Verification items for the finished model (mm, model axes). Face numbers are marked on the shaded views. A direction names the side the tool comes from. Round coordinates to 2 decimals unless told otherwise and drop trailing zeros. Loops run counter-clockwise (first coordinate to the right, second up) from the corner with the lowest first, then second, coordinate; pieces in that order, holes last. Notation, with made-up numbers: M 33.5,36 L 85.5,36 A20 cw 85.5,50 Z; hole C 26,58 d2. An arc over 180 degrees is marked long. One line per item, written item: value.
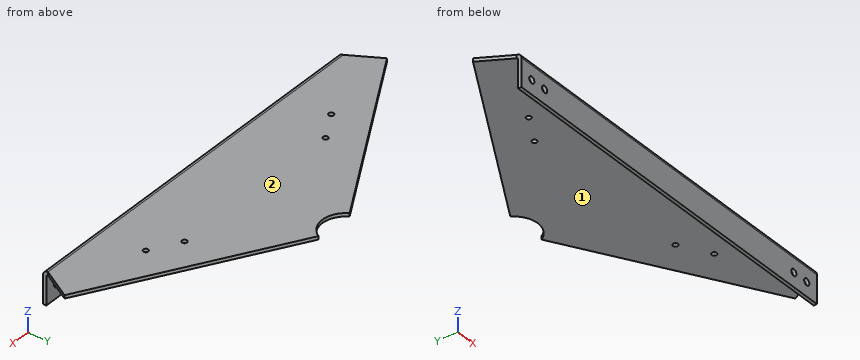
from build123d import *

# Parameters (mm, degrees)
SKETCH_10_R                   = 10
SM_BASE_FLANGE_3_DEPTH        = 2
SM_EDGE_FLANGE_6_DEPTH        = 230
SM_EDGE_FLANGE_6_BEND_DEPTH   = 230
SM_EDGE_FLANGE_6_BEND_2_DEPTH = 230
CUT_EXTRUDE_4_REACH           = 363.137
SKETCH_47_R                   = 2
CUT_EXTRUDE_6_REACH           = 263.424
SKETCH_50_R                   = 2
CUT_EXTRUDE_7_REACH           = 351.772
SKETCH_51_R                   = 2
CUT_EXTRUDE_8_REACH           = 349.61
SKETCH_52_R                   = 14
SKETCH_53_R                   = 1.5
CUT_EXTRUDE_9_DEPTH           = 10
OTHER_START                   = -20
OTHER_1_OUTLINE_R             = 1.5
OTHER_1_OUTLINE_R_2           = 10
OTHER_1_DEPTH                 = 20


# Read off the part's stored shape, not the designer's step: Полость1
# Sheet-metal steps are written as plain solids
with BuildPart() as part:
    # Эскиз10 → Базовая кромка3 (new body)
    with BuildSketch(Plane.XY):
        Polygon((0, 0), (-21, 36.373066959), (94, 235.558909829), (136, 235.558909829), (251, 36.373066959), (230, 0), align=None)
        with Locations((171.849364905, 123.465988394)):
            Circle(SKETCH_10_R, mode=Mode.SUBTRACT)
    extrude(amount=-SM_BASE_FLANGE_3_DEPTH)

    # Ребро-кромка6 section (across the edge) → Ребро-кромка6 (add)
    with BuildSketch(Plane(origin=(-21.866025404, 36.873066959, -2), x_dir=(0.8660254037844436, -0.4999999999999914, -3.4914813388431334e-15), z_dir=(0.4999999999999914, 0.8660254037844436, 0))):
        with BuildLine():
            Line((-2, 1), (-2, 18))
            Line((-2, 18), (0, 18))
            Line((0, 18), (0, 1))
            ThreePointArc((0, 1), (0.292893219, 0.292893219), (1, 0))
            Line((1, 0), (1, -2))
            ThreePointArc((1, -2), (-1.121320344, -1.121320344), (-2, 1))
        make_face()
    extrude(amount=SM_EDGE_FLANGE_6_DEPTH)

    # Ребро-кромка6 section 2 (across the edge) → Ребро-кромка6 bend (add)
    with BuildSketch(Plane(origin=(136.866025404, 236.058909829, -2), x_dir=(-0.8660254037844363, -0.5000000000000041, -3.4914813388431334e-15), z_dir=(0.5000000000000041, -0.8660254037844363, 0))):
        with BuildLine():
            Line((-2, 1), (-2, 18))
            Line((-2, 18), (0, 18))
            Line((0, 18), (0, 1))
            ThreePointArc((0, 1), (0.292893219, 0.292893219), (1, 0))
            Line((1, 0), (1, -2))
            ThreePointArc((1, -2), (-1.121320344, -1.121320344), (-2, 1))
        make_face()
    extrude(amount=SM_EDGE_FLANGE_6_BEND_DEPTH)

    # Ребро-кромка6 section 3 (across the edge) → Ребро-кромка6 bend 2 (add)
    with BuildSketch(Plane(origin=(230, -1, -2), x_dir=(0, 1, 0), z_dir=(-1, 0, 0))):
        with BuildLine():
            Line((-2, 1), (-2, 18))
            Line((-2, 18), (0, 18))
            Line((0, 18), (0, 1))
            ThreePointArc((0, 1), (0.292893219, 0.292893219), (1, 0))
            Line((1, 0), (1, -2))
            ThreePointArc((1, -2), (-1.121320344, -1.121320344), (-2, 1))
        make_face()
    extrude(amount=SM_EDGE_FLANGE_6_BEND_2_DEPTH)

    # Эскиз47 → Вырез-Вытянуть4 (cut, up to next)
    with BuildSketch(Plane(origin=(-34.098076211, 19.686533479, 0), x_dir=(0, 0, 1), z_dir=(-0.866025403784443, 0.4999999999999925, 3.788649256556814e-15)), mode=Mode.PRIVATE) as cut_extrude_4_sk1:
        with Locations(Location((-11.5, 29, 0), (0, 0, 270))):
            Circle(SKETCH_47_R)
    cut_extrude_4_tool1 = extrude(cut_extrude_4_sk1.sketch, amount=-CUT_EXTRUDE_4_REACH, mode=Mode.PRIVATE) & part.part
    # Эскиз47 → Вырез-Вытянуть4 (cut, up to next)
    with BuildSketch(Plane(origin=(-34.098076211, 19.686533479, 0), x_dir=(0, 0, 1), z_dir=(-0.866025403784443, 0.4999999999999925, 3.788649256556814e-15)), mode=Mode.PRIVATE) as cut_extrude_4_sk2:
        with Locations(Location((-11.5, 39, 0), (0, 0, 270))):
            Circle(SKETCH_47_R)
    cut_extrude_4_tool2 = extrude(cut_extrude_4_sk2.sketch, amount=-CUT_EXTRUDE_4_REACH, mode=Mode.PRIVATE) & part.part
    # Эскиз47 → Вырез-Вытянуть4 (cut, up to next)
    with BuildSketch(Plane(origin=(-34.098076211, 19.686533479, 0), x_dir=(0, 0, 1), z_dir=(-0.866025403784443, 0.4999999999999925, 3.788649256556814e-15)), mode=Mode.PRIVATE) as cut_extrude_4_sk3:
        with Locations(Location((-11.5, 233, 0), (0, 0, 270))):
            Circle(SKETCH_47_R)
    cut_extrude_4_tool3 = extrude(cut_extrude_4_sk3.sketch, amount=-CUT_EXTRUDE_4_REACH, mode=Mode.PRIVATE) & part.part
    # Эскиз47 → Вырез-Вытянуть4 (cut, up to next)
    with BuildSketch(Plane(origin=(-34.098076211, 19.686533479, 0), x_dir=(0, 0, 1), z_dir=(-0.866025403784443, 0.4999999999999925, 3.788649256556814e-15)), mode=Mode.PRIVATE) as cut_extrude_4_sk4:
        with Locations(Location((-11.5, 243, 0), (0, 0, 270))):
            Circle(SKETCH_47_R)
    cut_extrude_4_tool4 = extrude(cut_extrude_4_sk4.sketch, amount=-CUT_EXTRUDE_4_REACH, mode=Mode.PRIVATE) & part.part
    add(cut_extrude_4_tool1.solids().sort_by_distance((-19.598076, 44.80127, -11.5))[0], mode=Mode.SUBTRACT)
    add(cut_extrude_4_tool2.solids().sort_by_distance((-14.598076, 53.461524, -11.5))[0], mode=Mode.SUBTRACT)
    add(cut_extrude_4_tool3.solids().sort_by_distance((82.401924, 221.470453, -11.5))[0], mode=Mode.SUBTRACT)
    add(cut_extrude_4_tool4.solids().sort_by_distance((87.401924, 230.130707, -11.5))[0], mode=Mode.SUBTRACT)

    # Эскиз50 → Вырез-Вытянуть6 (cut, up to next)
    with BuildSketch(Plane(origin=(206.598076211, 119.279454915, 0), x_dir=(0, 0, -1), z_dir=(0.866025403784436, 0.5000000000000047, 3.0623287353932815e-15)), mode=Mode.PRIVATE) as cut_extrude_6_sk1:
        with Locations(Location((11.5, -86, 0), (0, 0, 90))):
            Circle(SKETCH_50_R)
    cut_extrude_6_tool1 = extrude(cut_extrude_6_sk1.sketch, amount=-CUT_EXTRUDE_6_REACH, mode=Mode.PRIVATE) & part.part
    # Эскиз50 → Вырез-Вытянуть6 (cut, up to next)
    with BuildSketch(Plane(origin=(206.598076211, 119.279454915, 0), x_dir=(0, 0, -1), z_dir=(0.866025403784436, 0.5000000000000047, 3.0623287353932815e-15)), mode=Mode.PRIVATE) as cut_extrude_6_sk2:
        with Locations(Location((11.5, -76, 0), (0, 0, 90))):
            Circle(SKETCH_50_R)
    cut_extrude_6_tool2 = extrude(cut_extrude_6_sk2.sketch, amount=-CUT_EXTRUDE_6_REACH, mode=Mode.PRIVATE) & part.part
    # Эскиз50 → Вырез-Вытянуть6 (cut, up to next)
    with BuildSketch(Plane(origin=(206.598076211, 119.279454915, 0), x_dir=(0, 0, -1), z_dir=(0.866025403784436, 0.5000000000000047, 3.0623287353932815e-15)), mode=Mode.PRIVATE) as cut_extrude_6_sk3:
        with Locations(Location((11.5, 118, 0), (0, 0, 90))):
            Circle(SKETCH_50_R)
    cut_extrude_6_tool3 = extrude(cut_extrude_6_sk3.sketch, amount=-CUT_EXTRUDE_6_REACH, mode=Mode.PRIVATE) & part.part
    # Эскиз50 → Вырез-Вытянуть6 (cut, up to next)
    with BuildSketch(Plane(origin=(206.598076211, 119.279454915, 0), x_dir=(0, 0, -1), z_dir=(0.866025403784436, 0.5000000000000047, 3.0623287353932815e-15)), mode=Mode.PRIVATE) as cut_extrude_6_sk4:
        with Locations(Location((11.5, 128, 0), (0, 0, 90))):
            Circle(SKETCH_50_R)
    cut_extrude_6_tool4 = extrude(cut_extrude_6_sk4.sketch, amount=-CUT_EXTRUDE_6_REACH, mode=Mode.PRIVATE) & part.part
    add(cut_extrude_6_tool1.solids().sort_by_distance((249.598076, 44.80127, -11.5))[0], mode=Mode.SUBTRACT)
    add(cut_extrude_6_tool2.solids().sort_by_distance((244.598076, 53.461524, -11.5))[0], mode=Mode.SUBTRACT)
    add(cut_extrude_6_tool3.solids().sort_by_distance((147.598076, 221.470453, -11.5))[0], mode=Mode.SUBTRACT)
    add(cut_extrude_6_tool4.solids().sort_by_distance((142.598076, 230.130707, -11.5))[0], mode=Mode.SUBTRACT)

    # Эскиз51 → Вырез-Вытянуть7 (cut, up to next)
    with BuildSketch(Plane.XZ.offset(3), mode=Mode.PRIVATE) as cut_extrude_7_sk1:
        with Locations(Location((222, -11.5, 0), (0, 0, 270))):
            Circle(SKETCH_51_R)
    cut_extrude_7_tool1 = extrude(cut_extrude_7_sk1.sketch, amount=-CUT_EXTRUDE_7_REACH, mode=Mode.PRIVATE) & part.part
    # Эскиз51 → Вырез-Вытянуть7 (cut, up to next)
    with BuildSketch(Plane.XZ.offset(3), mode=Mode.PRIVATE) as cut_extrude_7_sk2:
        with Locations(Location((212, -11.5, 0), (0, 0, 270))):
            Circle(SKETCH_51_R)
    cut_extrude_7_tool2 = extrude(cut_extrude_7_sk2.sketch, amount=-CUT_EXTRUDE_7_REACH, mode=Mode.PRIVATE) & part.part
    # Эскиз51 → Вырез-Вытянуть7 (cut, up to next)
    with BuildSketch(Plane.XZ.offset(3), mode=Mode.PRIVATE) as cut_extrude_7_sk3:
        with Locations(Location((18, -11.5, 0), (0, 0, 270))):
            Circle(SKETCH_51_R)
    cut_extrude_7_tool3 = extrude(cut_extrude_7_sk3.sketch, amount=-CUT_EXTRUDE_7_REACH, mode=Mode.PRIVATE) & part.part
    # Эскиз51 → Вырез-Вытянуть7 (cut, up to next)
    with BuildSketch(Plane.XZ.offset(3), mode=Mode.PRIVATE) as cut_extrude_7_sk4:
        with Locations(Location((8, -11.5, 0), (0, 0, 270))):
            Circle(SKETCH_51_R)
    cut_extrude_7_tool4 = extrude(cut_extrude_7_sk4.sketch, amount=-CUT_EXTRUDE_7_REACH, mode=Mode.PRIVATE) & part.part
    add(cut_extrude_7_tool1.solids().sort_by_distance((222, -3, -11.5))[0], mode=Mode.SUBTRACT)
    add(cut_extrude_7_tool2.solids().sort_by_distance((212, -3, -11.5))[0], mode=Mode.SUBTRACT)
    add(cut_extrude_7_tool3.solids().sort_by_distance((18, -3, -11.5))[0], mode=Mode.SUBTRACT)
    add(cut_extrude_7_tool4.solids().sort_by_distance((8, -3, -11.5))[0], mode=Mode.SUBTRACT)

    # Эскиз52 → Вырез-Вытянуть8 (cut, up to next)
    with BuildSketch(Plane(origin=(0, 0, -2), x_dir=(-1, 0, 0), z_dir=(0, 0, -1)), mode=Mode.PRIVATE) as cut_extrude_8_sk1:
        with Locations((-115, 90.643992263)):
            Circle(SKETCH_52_R)
    cut_extrude_8_tool1 = extrude(cut_extrude_8_sk1.sketch, amount=-CUT_EXTRUDE_8_REACH, mode=Mode.PRIVATE) & part.part
    add(cut_extrude_8_tool1.solids().sort_by_distance((115, 90.643992, -2))[0], mode=Mode.SUBTRACT)

    # Эскиз53 → Вырез-Вытянуть9 (cut)
    with BuildSketch(Plane(origin=(0, 0, -2), x_dir=(-1, 0, 0), z_dir=(0, 0, -1))):
        with Locations((-40.121778265, 70.507041555)):
            Circle(SKETCH_53_R)
        with Locations((-22.801270189, 60.507041555)):
            Circle(SKETCH_53_R)
        with Locations((-60.121778265, 35.866025404)):
            Circle(SKETCH_53_R)
        with Locations((-42.801270189, 25.866025404)):
            Circle(SKETCH_53_R)
        with Locations((-95, 185.558909829)):
            Circle(SKETCH_53_R)
        with Locations((-95, 165.558909829)):
            Circle(SKETCH_53_R)
        with Locations((-135, 185.558909829)):
            Circle(SKETCH_53_R)
        with Locations((-135, 165.558909829)):
            Circle(SKETCH_53_R)
        with Locations((-207.198729811, 60.507041555)):
            Circle(SKETCH_53_R)
        with Locations((-189.878221735, 70.507041555)):
            Circle(SKETCH_53_R)
        with Locations((-187.198729811, 25.866025404)):
            Circle(SKETCH_53_R)
        with Locations((-169.878221735, 35.866025404)):
            Circle(SKETCH_53_R)
    extrude(amount=-CUT_EXTRUDE_9_DEPTH, mode=Mode.SUBTRACT)

    # Полость1 outline → Полость1 (cut)
    with BuildSketch(Plane.XY.offset(OTHER_START)):
        with BuildLine():
            Line((127.120094671, 83.636617208), (240.495741262, 18.17915713))
            Line((240.495741262, 18.17915713), (251, 36.373066959))
            Line((251, 36.373066959), (253.598076211, 37.873066959))
            Line((253.598076211, 37.873066959), (138.598076211, 237.058909829))
            Line((138.598076211, 237.058909829), (136, 235.558909829))
            Line((136, 235.558909829), (94, 235.558909829))
            Line((94, 235.558909829), (91.401923789, 237.058909829))
            Line((91.401923789, 237.058909829), (-23.598076211, 37.873066959))
            Line((-23.598076211, 37.873066959), (-21, 36.373066959))
            Line((-21, 36.373066959), (-10.495741262, 18.17915713))
            Line((-10.495741262, 18.17915713), (102.879905329, 83.636617208))
            ThreePointArc((102.879905329, 83.636617208), (115, 104.643992263), (127.120094671, 83.636617208))
        make_face()
        with Locations((22.801270189, 60.507041555)):
            Circle(OTHER_1_OUTLINE_R, mode=Mode.SUBTRACT)
        with Locations((40.121778265, 70.507041555)):
            Circle(OTHER_1_OUTLINE_R, mode=Mode.SUBTRACT)
        with Locations((189.878221735, 70.507041555)):
            Circle(OTHER_1_OUTLINE_R, mode=Mode.SUBTRACT)
        with Locations((207.198729811, 60.507041555)):
            Circle(OTHER_1_OUTLINE_R, mode=Mode.SUBTRACT)
        with Locations((171.849364905, 123.465988394)):
            Circle(OTHER_1_OUTLINE_R_2, mode=Mode.SUBTRACT)
        with Locations((95, 165.558909829)):
            Circle(OTHER_1_OUTLINE_R, mode=Mode.SUBTRACT)
        with Locations((95, 185.558909829)):
            Circle(OTHER_1_OUTLINE_R, mode=Mode.SUBTRACT)
        with Locations((135, 165.558909829)):
            Circle(OTHER_1_OUTLINE_R, mode=Mode.SUBTRACT)
        with Locations((135, 185.558909829)):
            Circle(OTHER_1_OUTLINE_R, mode=Mode.SUBTRACT)
    extrude(amount=OTHER_1_DEPTH, mode=Mode.SUBTRACT)


solid = part.part
(1) Sectioned sample at A-A on x = 105.5. Enter the section's corners in (y, z).
Completed:
outline: M -3,-20 L -1,-20 L -1,-3 A1 cw 0,-2 L 80.36,-2 L 80.36,0 L 0,0 A3 ccw -3,-3 Z
(2) Sectioned sample at B-B on y = 44.5. Enter the section's corners in (x, z), and give its area (3 significant figures).
Completed:
outline: M 35.09,-2 L 194.91,-2 L 194.91,0 L 35.09,0 Z
area: 320 mm^2
(3) Thickness scan on L1, parallel to X at y = -1.65, z = -11.5; L2, parallel to Y at x = 170, z = -12; L3, parallel to Z at x = 129.5, y = 33. Record the ranges inside material, lowest first. Write a range as from..to.
Completed:
L1: x = 0..6, 10..16, 20..210, 214..220, 224..230
L2: y = -3..-1
L3: z = -2..0
(4) Depth check by flat-ended pin: pin 1 Ø0.9 at (y, z) = (-1, -13) entering from +X; pin 2 Ø5 at (x, y) = (94.5, 64.5) entering from -Z; pin 3 Ø5 at (x, z) = (8, -11.5) entering from +Y. Enter the tip coordinate at first touch or a pass-through.
Completed:
pin 1: stops at x = 230
pin 2: stops at z = -2
pin 3: stops at y = -1
(5) Sectioned sample at D-D on y = 62. Enter the section's corners in (x, z), and give its area (3 significant figures).
Completed:
outline: M 65.4,-2 L 164.6,-2 L 164.6,0 L 65.4,0 Z
area: 198 mm^2
(6) Sectioned sample at C-C on x = 178.5. Enter the section's corners in (y, z), and give its area (3 significant figures).
Completed:
outline: M -3,-20 L -1,-20 L -1,-3 A1 cw 0,-2 L 53.97,-2 L 53.97,0 L 0,0 A3 ccw -3,-3 Z
area: 148 mm^2
(7) Tool access check on the marked faces 1 and 2. Record the directions out of +Z, -Z, +X, -X, +Y, -Y that give a thin tool (end or side, any length) a straight path to the whole face; none if there is none.
Completed:
face 1: -Z, +X, -X, +Y
face 2: +Z, +X, -X, +Y, -Y
